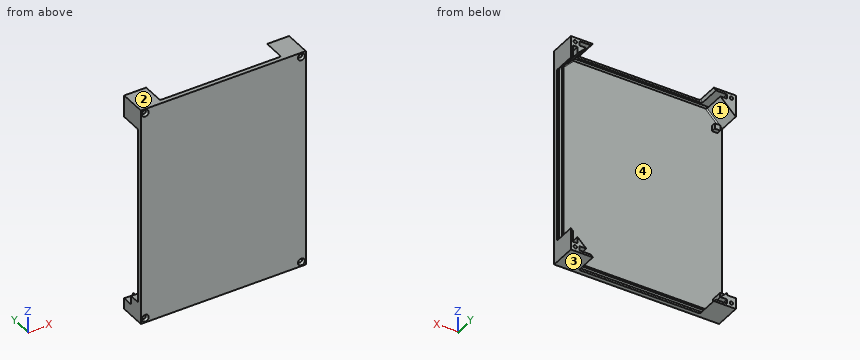
Autodesk Inventor part; units mm, degrees
ref_plane "Pracovní rovina2" through (0, 14, 0) normal (0, 1, 0) x (1, 0, 0)
ref_plane "Pracovní rovina3" through (0, 14, 0) normal (0, 1, 0) x (1, 0, 0)
ref_plane "YZ Plane" through (0, 0, 0) normal (1, 0, 0) x (0, 1, 0)
sketch "Náčrt1" plane through (0, 0, 0) normal (0, 1, 0) x (-1, 0, 0)
  line L0 (75, 100) -> (-75, 100)
  line L1 (-75, 100) -> (-75, -100)
  line L2 (-75, -100) -> (75, -100)
  line L3 (75, -100) -> (75, 100)
  line L4 (105, 0) -> (-105, 0)
  line L5 (0, -140) -> (0, 140)
  point P0 (0, 0)
  dimension "d0" = 200
  dimension "d1" = 150
extrude "Vysunutí1" add sketch "Náčrt1" along normal blind 4
sketch "Náčrt2" plane through (0, 4, 0) normal (0, 1, 0) x (1, 0, 0)
  line L0 (-75, -100) -> (-75, -80)
  line L1 (-75, -100) -> (-55, -100)
  line L2 (-75, 100) -> (-75, -100)
  line L3 (-75, -100) -> (75, -100)
  line L4 (-67, -98) -> (-57, -98)
  line L5 (-61, -94) -> (-67, -94)
  line L6 (-67, -94) -> (-67, -98)
  line L7 (-55, -100) -> (-57, -98)
  line L8 (-61, -94) -> (-75, -80)
  line L9 (55, -100) -> (75, -100)
  line L10 (75, -100) -> (75, -80)
  line L11 (75, -100) -> (75, 100)
  line L12 (57, -98) -> (67, -98)
  line L13 (67, -98) -> (67, -94)
  line L14 (67, -94) -> (61, -94)
  line L15 (57, -98) -> (55, -100)
  line L16 (69, -92) -> (73, -92)
  line L17 (73, -92) -> (73, -82)
  line L18 (69, -86) -> (69, -92)
  line L19 (75, -80) -> (73, -82)
  line L20 (69, -86) -> (61, -94)
  point P0 (0, 0)
  point P1 (55, -100)
  dimension "d4" = 20
  dimension "d17" = 4
  dimension "d18" = 2
  dimension "d19" = 8
  dimension "d20" = 10
  dimension "d21" = 6
  dimension "d66" = 20
  dimension "d67" = 20
  dimension "d70" = 2
  dimension "d71" = 10
  dimension "d72" = 8
  dimension "d74" = 4
  dimension "d75" = 6
  dimension "d77" = 10
  dimension "d78" = 2
  dimension "d79" = 8
  dimension "d80" = 4
  dimension "d81" = 6
extrude "Vysunutí7" add sketch "Náčrt2" along normal blind 20
mirror "Zrcadlit5" about plane through (0, 0, 0) normal (0, 0, 1) of "Vysunutí7"
ref_plane "Pracovní rovina2" through (0, 14, 0) normal (0, 1, 0) x (1, 0, 0)
sketch "Náčrt11" plane through (0, 0, 0) normal (0, -1, 0) x (1, 0, 0)
  line L0 (75, -100) -> (-75, -100)
  line L1 (-75, -100) -> (-75, 100)
  point P0 (0, 0)
  point P1 (-71, -96)
  dimension "d100" = 4
  dimension "d101" = 4
hole "Díra4" at (-71, 0, -96) direction (0, 1, 0) diameter 3 end through all countersink diameter 6.3 countersink angle 90
pattern_circular "Kruhové pole1" count 2 over 360 about axis through (0, -10, 0) along (0, 1, 0) of "Díra4"
mirror "Zrcadlit6" about plane through (0, 0, 0) normal (0, 0, 1) of "Kruhové pole1", "Díra4"
sketch "Náčrt12" plane through (0, 4, 0) normal (0, 1, 0) x (1, 0, 0)
  line L0 (-67, -98) -> (67, -98)
  line L1 (67, -98) -> (67, -94)
  line L2 (67, -94) -> (-67, -94)
  line L3 (-67, -94) -> (-67, -98)
  line L4 (-67, -98) -> (-67, -94)
  line L5 (67, -94) -> (67, -98)
  line L6 (61, -94) -> (67, -94)
  line L7 (67, -98) -> (57, -98)
  point P0 (0, 0)
extrude "Vysunutí9" cut sketch "Náčrt12" against normal blind 2
mirror "Zrcadlit7" about plane through (0, 0, 0) normal (0, 0, 1) of "Vysunutí9"
sketch "Náčrt13" plane through (0, 4, 0) normal (0, 1, 0) x (1, 0, 0)
  line L0 (69, -92) -> (73, -92)
  line L1 (73, -92) -> (73, 92)
  line L2 (73, 92) -> (69, 92)
  line L3 (69, 92) -> (69, -92)
  line L4 (73, -92) -> (69, -92)
  line L5 (73, 92) -> (69, 92)
  line L6 (73, 82) -> (73, 92)
  line L7 (69, 92) -> (69, 86)
  point P0 (0, 0)
extrude "Vysunutí10" cut sketch "Náčrt13" against normal blind 2
sketch "Náčrt14" plane through (0, 4, 0) normal (0, 1, 0) x (1, 0, 0)
  line L0 (-71, -80) -> (-66, -80)
  line L1 (-66, -80) -> (-66, -75)
  line L2 (-66, -75) -> (-71, -75)
  line L3 (-71, -75) -> (-71, -80)
  line L4 (-75, 80) -> (-75, -80)
  line L5 (-75, -100) -> (-55, -100)
  point P0 (0, 0)
  dimension "d116" = 5
  dimension "d117" = 5
  dimension "d118" = 4
  dimension "d119" = 20
extrude "Vysunutí11" add sketch "Náčrt14" along normal blind 4
fillet "Zaoblení1" radius 1 9 edges at (-56, 4, -99) (56, 4, -99) (65, 4, -90) (74, 4, -81) (-56, 4, 99) (-68, 4, 87) (65, 4, 90) (74, 4, 81) (56, 4, 99)
sketch "Náčrt15" plane through (-75, 24, -100) normal (0, 1, 0) x (1, 0, 0)
  line L0 (0, -10) -> (8, -10)
  line L1 (8, -10) -> (8, -20)
  line L2 (8, -20) -> (0, -20)
  line L3 (0, -20) -> (0, -10)
  line L4 (0, -20) -> (0, 0)
  point P0 (75, -100)
  dimension "d123" = 8
  dimension "d124" = 10
extrude "Vysunutí12" cut sketch "Náčrt15" against normal up to surface (20 mm away)
sketch "Náčrt16" plane through (0, 4, 0) normal (0, 1, 0) x (1, 0, 0)
  line L0 (-75, 90) -> (-75, -78.5858)
  line L1 (-75, 90) -> (-67, 90)
  line L2 (-67, 90) -> (-67, 82)
  line L3 (-67, 82) -> (-75, 82)
  line L4 (-75, 82) -> (-75, 90)
  line L5 (-75, 90) -> (-67, 90)
  line L6 (-67, 90) -> (-67, 88)
  point P0 (0, 0)
  dimension "d142" = 8
ref_plane "Pracovní rovina3" through (0, 14, 0) normal (0, 1, 0) x (1, 0, 0)
extrude "Vysunutí14" add sketch "Náčrt16" along normal blind 10
sketch "Náčrt18" plane through (0, 14, 0) normal (0, 1, 0) x (1, 0, 0)
  line L0 (-67, 82) -> (-67, 88)
  line L1 (-75, 82) -> (-67, 82)
  point P0 (0, 0)
  point P1 (-69.5, 86)
  dimension "d145" = 2.5
  dimension "d146" = 4
hole "Díra6" at (-69.5, 14, -86) direction (0, -1, 0) diameter 3 depth 5
properties part number "Cabinet"
Geometry check sheet. Reference: the model listing, model coordinates, mm. Face numbers are marked on the shaded views. A direction names the side the tool comes from. Give positions to 0.01 mm unless a question says otherwise; leave off trailing zeros. Order: outer loops, then holes, each group sorted by start corner. A loop starts at its lowest first (then second) coordinate and runs counter-clockwise, first axis right, second up. Notation, with made-up numbers: (83, -37) -> (129, -37) arc R18 cw to (129, -8) -> close; hole circle Ø5 at (-0.5, -14.5). An arc over 180 degrees is marked (long way). Write each question's results on one line, items separated by ' | '. Start each with the question number.
(1) Sectioned sample at A-A (y = 20.75). Give the number of separate pieces and of enclosed holes in the cut face, plus the area to 3 significant figures.
(2) Scan lines: line 1 (Z direction, x = 71, y = 7.25); line 2 (X direction, y = 10, z = 96); line 3 (Z direction, x = -65, y = 12). Record each from-to range of solid material in increasing order.
(3) Gauge pin test, flat ends, axial feed: P1, Ø8, axis at y = 15.5, z = -73.5, coming from the -X side; P2, Ø4, axis at x = 42.5, z = 10.5, coming from the +Y side; P3, Ø3.5, axis at x = -69.5, z = -86, coming from the -Y side; P4, Ø2.5, axis at x = -70.5, z = -87.5, coming from the +Y side. Record the tip position at first contact, or that the pin passes through.
(4) Access from +Z, -Z, +X, -X, +Y, -Y to the whole of each face (thin tool, end or side, straight path). Record for the marked faces 1 and 2.
(5) Sectioned sample at C-C (x = 35.5). Enter the section's corners in (y, z).
(6) Sectioned sample at B-B (z = -3.5). Enter the section's corners in (x, y), plus the area to 3 significant figures.
(7) Mould release check, pull along X, two halves, no side actions. Record for the marked faces 3 and 4: pulls with the +X half, pulls with the -X half, needs draft (parallel to the pull), parting line crosses it, or undercut.
Answer below:
1) separate pieces: 4 | enclosed holes: 4 | area: 532 mm2
2) line 1: -100 to -97.5, -94.5 to -92, 92 to 94.5, 97.5 to 100 | line 2: -75 to -72.5, -69.5 to -67, 67 to 69.5, 72.5 to 75 | line 3: -100 to -98, -94 to -90, 90 to 94, 98 to 100
3) P1: through | P2: y = 4 | P3: y = 0 | P4: y = 14
4) face 1: +Y | face 2: +Z, +X, -X, +Y, -Y
5) outline: (0, -100) -> (4, -100) -> (4, -98) -> (2, -98) -> (2, -94) -> (4, -94) -> (4, 94) -> (2, 94) -> (2, 98) -> (4, 98) -> (4, 100) -> (0, 100) -> close
6) outline: (-75, 0) -> (75, 0) -> (75, 4) -> (73, 4) -> (73, 2) -> (69, 2) -> (69, 4) -> (-75, 4) -> close | area: 592 mm2
7) face 3: needs draft | face 4: undercut
